Check sheet for the modelled part. Datum: model origin and axes. Units: mm. A direction names the side the tool comes from. Coordinates: 2 decimals unless noted, no trailing zeros. Loops run counter-clockwise (first coordinate to the right, second up) from the corner with the lowest first, then second, coordinate; pieces in that order, holes last. Notation, with made-up numbers: (87, 81.25) -> (91, 81.25) arc R18 cw to (91, 100.25) -> close; hole circle Ø1 at (74.5, -10). An arc over 180 degrees is marked (long way). Use CSV: the item, a comma, the result in double quotes. Start each with the question number.
1. Release check for a two-part mould opening along Z. For faces 6 (the face through (11.5, 10, -0.2)), 7 (the face through (-34.93, 152.987, -0.632)), 8 (the face through (-34.93, 126.153, 1.826)) record: pulls with the +Z half, pulls with the -Z half, needs draft (parallel to the pull), parting line crosses it, or undercut.
2. Thickness scan on L1, parallel to Z at x = 0, y = 5; L2, parallel to Y at x = 2.5, z = -13; L3, parallel to Z at x = -36, y = 15. Record the ranges inside material, lowest first.
3. Sectioned sample at D-D, the plane z = 9.5. Record the cut outline in (x, y).
4. Sectioned sample at B-B, the plane y = 137. Record the cut outline in (x, z), and give its area (3 significant figures).
5. Sectioned sample at C-C, the plane x = 0. Record the cut outline in (y, z).
6. Sectioned sample at A-A, the plane z = 0. Record the cut outline in (x, y), and give its area (3 significant figures).
7. Gauge pin test, flat ends, axial feed: pin 1 (1 mm diameter, centred on y = 54.5, z = 6.5, fed in from +X); pin 2 (13 mm diameter, centred on x = 7.5, z = -3, fed in from +Y); pin 3 (12.5 mm diameter, centred on x = -26.5, y = 59.5, fed in from -Z); pin 4 (7.5 mm diameter, centred on x = -31.5, y = 85, fed in from +Z). Record the tip position at first contact, or that the pin passes through.
8. Set-up check for faces 1 (the face through (-40, 92, 1)), 2 (the face through (-30, 96, 1)), 3 (the face through (-2, 0, 11)), 4 (the face through (-33, 62, 5)), 5 (the face through (-33, 62, -5)): record each of +Z, -Z, +X, -X, +Y, -Y from which the full face is reachable in a straight line by a thin tool's end or side.
Autodesk Inventor part; units mm, degrees
ref_plane "YZ Plane" through (0, 0, 0) normal (1, 0, 0) x (0, 1, 0)
ref_plane "XZ Plane" through (0, 0, 0) normal (0, 1, 0) x (-1, 0, 0)
ref_plane "XY Plane" through (0, 0, 0) normal (0, 0, 1) x (1, 0, 0)
sketch "Szkic2" plane through (0, 0, 0) normal (0, 1, 0) x (-1, 0, 0)
  circle A0 centre (0, 0) radius 11
  circle A1 centre (0, 0) radius 16
  dimension "d0" = 22
  dimension "d1" = 5
extrude "Wyciągnięcie proste1" add sketch "Szkic2" along normal blind 10
sketch "Szkic4" plane through (0, 0, 0) normal (0, 0, 1) x (1, 0, 0)
  line L0 (0, 0) -> (-30, 0)
  line L1 (-30, 0) -> (-30, 10)
  line L2 (-30, 10) -> (0, 10)
  line L3 (0, 10) -> (0, 0)
  line L4 (-30, 0) -> (-40, 0)
  line L5 (-40, 0) -> (-40, 137)
  line L6 (-40, 137) -> (-30, 137)
  line L7 (-30, 137) -> (-30, 0)
  point P0 (-30, 10)
  dimension "d7" = 137
  dimension "d8" = 30
  dimension "d9" = 10
  dimension "d10" = 10
extrude "Wyciągnięcie proste2" add sketch "Szkic4" along normal mid plane 10
fillet "Zaokrąglenie1" radius 20 2 edges at (-40, 0, 0) (-30, 10, 0)
sketch "Szkic7" plane through (-30, 137, 5) normal (1, 0, 0) x (0, 0, -1)
  line L0 (10, 0) -> (0, 0)
  circle A0 centre (5, 0) radius 11
  circle A1 centre (5, 0) radius 16
  point P0 (5, -137)
  dimension "d14" = 22
  dimension "d15" = 32
extrude "Wyciągnięcie proste3" add sketch "Szkic7" against normal blind 10
sketch "Szkic8" plane through (0, 10, 0) normal (0, 1, 0) x (1, 0, 0)
  circle A0 centre (0, 0) radius 11
extrude "Wyciągnięcie proste4" cut sketch "Szkic8" against normal blind 10
sketch "Szkic9" plane through (-30, 30, 5) normal (1, 0, 0) x (0, 0, -1)
  line L0 (10, 107) -> (0, 107)
  circle A0 centre (5, 107) radius 11
  point P0 (5, -30)
extrude "Wyciągnięcie proste5" cut sketch "Szkic9" against normal blind 10
sketch "Szkic10" plane through (0, 10, 0) normal (0, -1, 0) x (1, 0, 0)
  circle A0 centre (0, 0) radius 11
extrude "Wyciągnięcie proste6" cut sketch "Szkic10" against normal blind 10
properties part number "Gora-dol-ramie"
Completed:
1,face 6,"needs draft"
1,face 7,"parting line crosses it"
1,face 8,"undercut"
2,L1,"-16 to -11, 11 to 16"
2,L2,"0 to 10"
2,L3,"-5 to 5"
3,outline,"(-40, 124.13) -> (-30, 124.13) -> (-30, 131.45) -> (-40, 131.45) -> close; (-40, 142.55) -> (-30, 142.55) -> (-30, 149.87) -> (-40, 149.87) -> close; (-12.87, 0) -> (-5.55, 0) -> (-5.55, 10) -> (-10, 10) arc R20 cw to (-12.87, 10.21) -> close; (5.55, 0) -> (12.87, 0) -> (12.87, 10) -> (5.55, 10) -> close"
4,outline,"(-40, -16) -> (-30, -16) -> (-30, -11) -> (-40, -11) -> close; (-40, 11) -> (-30, 11) -> (-30, 16) -> (-40, 16) -> close"
4,area,"100 mm²"
5,outline,"(0, -16) -> (10, -16) -> (10, -11) -> (0, -11) -> close; (0, 11) -> (10, 11) -> (10, 16) -> (0, 16) -> close"
6,outline,"(-40, 20) arc R20 ccw to (-20, 0) -> (-11, 0) -> (-11, 10.03) arc R20 cw to (-30, 30) -> (-30, 126) -> (-40, 126) -> close; (-40, 148) -> (-30, 148) -> (-30, 153) -> (-40, 153) -> close; (11, 0) -> (16, 0) -> (16, 10) -> (11, 10) -> close"
6,area,"1,550 mm²"
7,pin 1,"through"
7,pin 2,"y = 10"
7,pin 3,"z = -5"
7,pin 4,"z = 5"
8,face 1,"+Z, -Z, -X, +Y, -Y"
8,face 2,"+Z, -Z, +X, +Y"
8,face 3,"+Z, -Z, +X, -X, -Y"
8,face 4,"+Z, -X, -Y"
8,face 5,"-Z, -X, -Y"
